Input: dimensioned drawing with shaded views. Units: mm. Origin: part minimum x, y, z. Give positions to 0.01 mm unless a question says otherwise; leave off trailing zeros. Loops run counter-clockwise (first coordinate to the right, second up) from the corner with the lowest first, then second, coordinate; pieces in that order, holes last. Notation, with made-up numbers: M -8,-6.5 L 20,-6.5 A19 ccw 20,-2.5 Z; hole C -0.75,-13.75 d8. An arc over 180 degrees is marked long. Answer in a Markdown table with one row per item.
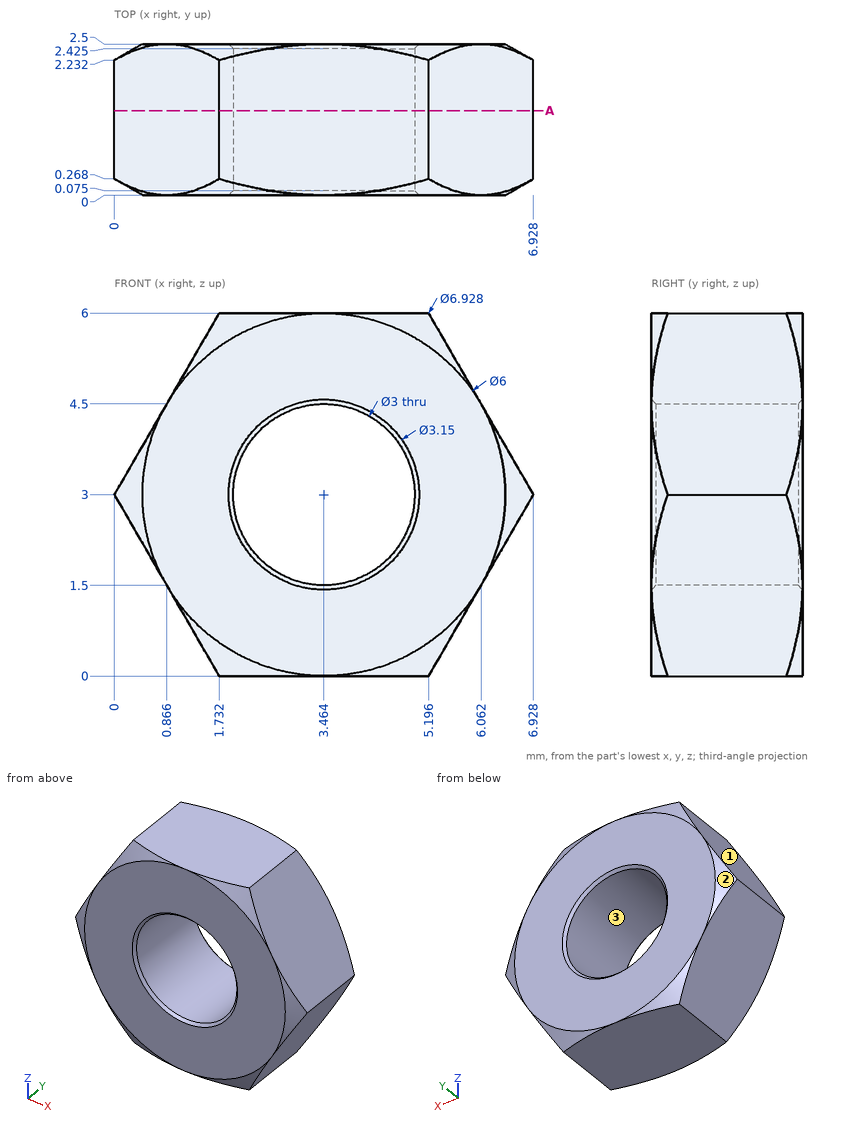
Q1. Contact query for a flat-ended pin moving along its axis: pin 1 Ø1.8 at (x, z) = (3.46, 3) entering from -Y. Output: stop coordinate, or through.
Values follow:
| item | result |
|---|---|
| pin 1 | through |
Q2. Mould query, pull axis Z, two halves, no side actions, for the marked faces 1, 2 and 3. Classes: +Z half, -Z half, draft (parallel to the pull), parting line (faces both ways), or undercut.
Values follow:
| item | result |
|---|---|
| face 1 | +Z half |
| face 2 | parting line |
| face 3 | undercut |
Q3. Ray query, probe 1 along Z at (x, y) = (2.5, 2.25); probe 2 along Z at (x, y) = (4.25, 1.95); probe 3 along X at (y, z) = (2.15, 4.25) (1 decimal). Return the intervals inside material, ascending. Write a range as from..to.
Values follow:
| item | result |
|---|---|
| probe 1 | 0..1.85, 4.15..6 |
| probe 2 | 0..1.72, 4.28..6 |
| probe 3 | 0.7..2.6, 4.3..6.2 |
Q4. Section query A-A (y = 1.4). Output: boundary loops of the cut face in (x, z), plus the area to 3 significant figures.
Values follow:
| item | result |
|---|---|
| outline | M 0,3 L 1.73,0 L 5.2,0 L 6.93,3 L 5.2,6 L 1.73,6 Z; hole C 3.46,3 d3 |
| area | 24.1 mm^2 |
